CAD build for the part. Positions are in the model's coordinates, mm. A direction names the side the tool comes from. Give positions to 0.01 mm unless a question says otherwise; leave off trailing zeros. Write each loop counter-clockwise with the first axis right and the second up, starting at its lowest first coordinate (ties: lowest second). Pieces come first, ordered by that corner, then holes. Notation, with made-up numbers: (-29, 63.25) - (7, 63.25) arc R14 ccw to (7, 71.25) - close; hole circle Ø9 at (55.25, -24). An arc over 180 degrees is marked (long way). Put each result on its own line as item: value. Start each with the question number.
1. Mould opens along X. For faces 6 (the flat face through (125, 1, 1)), 7 (the flat face through (-57, -3, 20)), 8 (the flat face through (-125, 1, 1)) say: +X half, -X half, draft (parallel to the pull), parting line (faces both ways), or undercut.
2. Cut at A-A on x = -24. List the corners of the cut face in (y, z).
3. Cut at B-B on z = -43.5. List the corners of the cut face in (x, y).
4. Tool access for faces 1 (the flat face through (-2, 3, -1)), 2 (the flat face through (-2, 0, 0)), 3 (the cylindrical face through (-122.15, 1.52, 46.99)), 4 (the flat face through (-2, 0, 37)), 5 (the flat face through (-2, 0, -38)): list every direction of +Z, -Z, +X, -X, +Y, -Y with a clear straight run to the whole face (end or side of a thin tool).
5. Wall check: line 1 (X direction, y = 0.75, z = 29.33) (3 decimals); line 2 (Z direction, x = 40, y = 1.05) (3 decimals); line 3 (Y direction, x = -108, z = -42). Give the ranges that are in metal, low to high.
6. Drop flat-ended pins along their axis: pin 1 (12.5 mm diameter, centred on x = 44, z = 37.5, fed in from -Y); pin 2 (1.5 mm diameter, centred on x = -81.5, y = -1, fed in from +Z); pin 3 (1 mm diameter, centred on x = 12, y = -2.5, fed in from -Z). Give the stop position or say it passes through.
from build123d import *

# Parameters (mm, degrees)
SKETCH_1_W          = 250
SKETCH_1_H          = 100
EXTRUDE_1_DEPTH     = 3
FILLET_1_R          = 10
SKETCH_2_R          = 1.525
CUT_EXTRUDE_1_DEPTH = 3
SKETCH_3_R          = 1.525
CUT_EXTRUDE_2_DEPTH = 3
SKETCH_4_W          = 250
SKETCH_4_H          = 6
EXTRUDE_2_DEPTH     = 6
FILLET_2_R          = 2
CUT_EXTRUDE_3_REACH = 11
SKETCH_5_R          = 1.7
CUT_EXTRUDE_4_REACH = 11
SKETCH_6_R          = 1.7
SKETCH_7_W          = 13
SKETCH_7_H          = 10
CUT_EXTRUDE_5_DEPTH = 3
FILLET_3_R          = 2


with BuildPart() as part:
    # 草图1 → 凸台-拉伸1 (new body)
    with BuildSketch(Plane(origin=(0, 0, 0), x_dir=(1, 0, 0), z_dir=(0, 1, 0))):
        Rectangle(SKETCH_1_W, SKETCH_1_H)
    extrude(amount=EXTRUDE_1_DEPTH)

    # 圆角1
    fillet_1_edges = [part.edges().sort_by_distance(p)[0] for p in [
        (125, 1.5, 50),
        (-125, 1.5, 50),
        (-125, 1.5, -50),
        (125, 1.5, -50),
    ]]
    fillet(fillet_1_edges, radius=FILLET_1_R)

    # 草图2 → 切除-拉伸1 (cut)
    with BuildSketch(Plane(origin=(0, 3, 0), x_dir=(1, 0, 0), z_dir=(0, 1, 0))):
        with Locations((-117.5, 32.5)):
            Circle(SKETCH_2_R)
        with Locations((117.5, 32.5)):
            Circle(SKETCH_2_R)
        with Locations((117.5, -32.5)):
            Circle(SKETCH_2_R)
        with Locations((-117.5, -32.5)):
            Circle(SKETCH_2_R)
    extrude(amount=-CUT_EXTRUDE_1_DEPTH, mode=Mode.SUBTRACT)

    # 草图3 → 切除-拉伸2 (cut)
    with BuildSketch(Plane(origin=(0, 3, 0), x_dir=(1, 0, 0), z_dir=(0, 1, 0))):
        with Locations((-40, -29.33)):
            Circle(SKETCH_3_R)
        with Locations((40, -29.33)):
            Circle(SKETCH_3_R)
    extrude(amount=-CUT_EXTRUDE_2_DEPTH, mode=Mode.SUBTRACT)

    # 草图4 → 凸台-拉伸2 (add)
    with BuildSketch(Plane.XZ):
        with Locations((0, 20)):
            Rectangle(SKETCH_4_W, SKETCH_4_H)
        with Locations((0, -20)):
            Rectangle(SKETCH_4_W, SKETCH_4_H)
    extrude(amount=EXTRUDE_2_DEPTH)

    # 圆角2
    fillet_2_edges = [part.edges().sort_by_distance(p)[0] for p in [
        (0, 0, 17),
        (0, 0, 23),
        (-125, -6, 20),
        (0, -6, 17),
        (125, -6, 20),
        (0, -6, 23),
        (0, 0, -23),
        (0, 0, -17),
        (-125, -6, -20),
        (0, -6, -23),
        (125, -6, -20),
        (0, -6, -17),
    ]]
    fillet(fillet_2_edges, radius=FILLET_2_R)

    # 草图5 → 切除-拉伸3 (cut, up to next)
    with BuildSketch(Plane(origin=(0, 3, 0), x_dir=(1, 0, 0), z_dir=(0, 1, 0)), mode=Mode.PRIVATE) as cut_extrude_3_sk1:
        with Locations((-31.176914536, 18)):
            Circle(SKETCH_5_R)
    cut_extrude_3_tool1 = extrude(cut_extrude_3_sk1.sketch, amount=-CUT_EXTRUDE_3_REACH, mode=Mode.PRIVATE) & part.part
    add(cut_extrude_3_tool1.solids().sort_by_distance((-31.176915, 3, -18))[0], mode=Mode.SUBTRACT)
    # 草图5 → 切除-拉伸3 (cut, up to next)
    with BuildSketch(Plane(origin=(0, 3, 0), x_dir=(1, 0, 0), z_dir=(0, 1, 0)), mode=Mode.PRIVATE) as cut_extrude_3_sk2:
        with Locations((31.176914536, 18)):
            Circle(SKETCH_5_R)
    cut_extrude_3_tool2 = extrude(cut_extrude_3_sk2.sketch, amount=-CUT_EXTRUDE_3_REACH, mode=Mode.PRIVATE) & part.part
    add(cut_extrude_3_tool2.solids().sort_by_distance((31.176915, 3, -18))[0], mode=Mode.SUBTRACT)
    # 草图5 → 切除-拉伸3 (cut, up to next)
    with BuildSketch(Plane(origin=(0, 3, 0), x_dir=(1, 0, 0), z_dir=(0, 1, 0)), mode=Mode.PRIVATE) as cut_extrude_3_sk3:
        with Locations((-18, -31.176914536)):
            Circle(SKETCH_5_R)
    cut_extrude_3_tool3 = extrude(cut_extrude_3_sk3.sketch, amount=-CUT_EXTRUDE_3_REACH, mode=Mode.PRIVATE) & part.part
    add(cut_extrude_3_tool3.solids().sort_by_distance((-18, 3, 31.176915))[0], mode=Mode.SUBTRACT)
    # 草图5 → 切除-拉伸3 (cut, up to next)
    with BuildSketch(Plane(origin=(0, 3, 0), x_dir=(1, 0, 0), z_dir=(0, 1, 0)), mode=Mode.PRIVATE) as cut_extrude_3_sk4:
        with Locations((18, -31.176914536)):
            Circle(SKETCH_5_R)
    cut_extrude_3_tool4 = extrude(cut_extrude_3_sk4.sketch, amount=-CUT_EXTRUDE_3_REACH, mode=Mode.PRIVATE) & part.part
    add(cut_extrude_3_tool4.solids().sort_by_distance((18, 3, 31.176915))[0], mode=Mode.SUBTRACT)

    # 草图6 → 切除-拉伸4 (cut, up to next)
    with BuildSketch(Plane(origin=(0, 3, 0), x_dir=(1, 0, 0), z_dir=(0, 1, 0)), mode=Mode.PRIVATE) as cut_extrude_4_sk1:
        with Locations((-56.5, -5)):
            Circle(SKETCH_6_R)
    cut_extrude_4_tool1 = extrude(cut_extrude_4_sk1.sketch, amount=-CUT_EXTRUDE_4_REACH, mode=Mode.PRIVATE) & part.part
    add(cut_extrude_4_tool1.solids().sort_by_distance((-56.5, 3, 5))[0], mode=Mode.SUBTRACT)
    # 草图6 → 切除-拉伸4 (cut, up to next)
    with BuildSketch(Plane(origin=(0, 3, 0), x_dir=(1, 0, 0), z_dir=(0, 1, 0)), mode=Mode.PRIVATE) as cut_extrude_4_sk2:
        with Locations((56.5, -5)):
            Circle(SKETCH_6_R)
    cut_extrude_4_tool2 = extrude(cut_extrude_4_sk2.sketch, amount=-CUT_EXTRUDE_4_REACH, mode=Mode.PRIVATE) & part.part
    add(cut_extrude_4_tool2.solids().sort_by_distance((56.5, 3, 5))[0], mode=Mode.SUBTRACT)
    # 草图6 → 切除-拉伸4 (cut, up to next)
    with BuildSketch(Plane(origin=(0, 3, 0), x_dir=(1, 0, 0), z_dir=(0, 1, 0)), mode=Mode.PRIVATE) as cut_extrude_4_sk3:
        with Locations((-56.5, -45)):
            Circle(SKETCH_6_R)
    cut_extrude_4_tool3 = extrude(cut_extrude_4_sk3.sketch, amount=-CUT_EXTRUDE_4_REACH, mode=Mode.PRIVATE) & part.part
    add(cut_extrude_4_tool3.solids().sort_by_distance((-56.5, 3, 45))[0], mode=Mode.SUBTRACT)
    # 草图6 → 切除-拉伸4 (cut, up to next)
    with BuildSketch(Plane(origin=(0, 3, 0), x_dir=(1, 0, 0), z_dir=(0, 1, 0)), mode=Mode.PRIVATE) as cut_extrude_4_sk4:
        with Locations((56.5, -45)):
            Circle(SKETCH_6_R)
    cut_extrude_4_tool4 = extrude(cut_extrude_4_sk4.sketch, amount=-CUT_EXTRUDE_4_REACH, mode=Mode.PRIVATE) & part.part
    add(cut_extrude_4_tool4.solids().sort_by_distance((56.5, 3, 45))[0], mode=Mode.SUBTRACT)

    # 草图7 → 切除-拉伸5 (cut)
    with BuildSketch(Plane.XZ.offset(6)):
        with Locations((-56.5, 20)):
            Rectangle(SKETCH_7_W, SKETCH_7_H)
        with Locations((56.5, 20)):
            Rectangle(SKETCH_7_W, SKETCH_7_H)
    extrude(amount=-CUT_EXTRUDE_5_DEPTH, mode=Mode.SUBTRACT)

    # 圆角3
    fillet_3_edges = [part.edges().sort_by_distance(p)[0] for p in [
        (-63, -5.414213562, 22.414213562),
        (-50, -5.414213562, 22.414213562),
        (50, -5.414213562, 22.414213562),
        (63, -5.414213562, 22.414213562),
        (63, -3.5, 17),
        (63, -3.5, 23),
        (63, -5.414213562, 17.585786438),
        (50, -3.5, 17),
        (50, -3.5, 23),
        (50, -5.414213562, 17.585786438),
        (63, -6, 20),
        (50, -6, 20),
        (-50, -3.5, 17),
        (-50, -3.5, 23),
        (-50, -5.414213562, 17.585786438),
        (-63, -3.5, 17),
        (-63, -3.5, 23),
        (-63, -5.414213562, 17.585786438),
        (-50, -6, 20),
        (-63, -6, 20),
    ]]
    fillet(fillet_3_edges, radius=FILLET_3_R)


solid = part.part
Report:
1. face 6: +X half
1. face 7: undercut
1. face 8: -X half
2. outline: (-6, -21) arc R2 ccw to (-4, -23) - (-2, -23) arc R2 cw to (0, -25) - (0, -50) - (3, -50) - (3, 50) - (0, 50) - (0, 25) arc R2 cw to (-2, 23) - (-4, 23) arc R2 ccw to (-6, 21) - (-6, 19) arc R2 ccw to (-4, 17) - (-2, 17) arc R2 cw to (0, 15) - (0, -15) arc R2 cw to (-2, -17) - (-4, -17) arc R2 ccw to (-6, -19) - close
3. outline: (-124.37, 0) - (124.37, 0) - (124.37, 3) - (-124.37, 3) - close
4. face 1: +Z, -Z, +X, -X, +Y
4. face 2: +X, -X, -Y
4. face 3: +Z, -X, +Y, -Y
4. face 4: +Z, +X, -X, -Y
4. face 5: -Z, +X, -X, -Y
5. line 1: x = -125 to -41.525, -38.475 to 38.475, 41.525 to 125
5. line 2: z = -50 to 27.805, 30.855 to 50
5. line 3: y = 0 to 3
6. pin 1: stops at y = 0
6. pin 2: stops at z = 24.03
6. pin 3: stops at z = -23
